Here's how the part is built. I have some questions about the finished solid (model axes, mm). A direction names the side the tool comes from. Give positions to 0.01 mm unless a question says otherwise; leave off trailing zeros. Loops run counter-clockwise (first coordinate to the right, second up) from the corner with the lowest first, then second, coordinate; pieces in that order, holes last. Notation, with made-up numbers: (-14, 79.5) - (12, 79.5) arc R35 cw to (12, 113.5) - close; hole circle Ø4 at (80, -21). An arc over 180 degrees is marked (long way). Use one line per item in the form item = value.
from build123d import *

# Parameters (mm, degrees)
BOSS_EXTRUDE1_DEPTH      = 5
BOSS_EXTRUDE1_DEPTH_BACK = 5
SKETCH1_R                = 1.75
SKETCH4_R                = 5.3
SKETCH4_R_2              = 1.75
BOSS_EXTRUDE2_DEPTH      = 1
M3_CLEARANCE_HOLE1_D     = 3.6


with BuildPart() as part:
    # Sketch1 → Boss-Extrude1 (new, two sides: drawn at the far end of the back side and taken through both)
    with BuildSketch(Plane.XY.offset(-BOSS_EXTRUDE1_DEPTH_BACK)):
        with BuildLine():
            Line((-29.2, 10.8), (-30.316718427, 10.8))
            ThreePointArc((-30.316718427, 10.8), (-35.8, 10), (-30.316718427, 9.2))
            Line((-30.316718427, 9.2), (-29.2, 9.2))
            Line((-29.2, 9.2), (-29.2, 10.8))
        make_face()
        with Locations(Location((-33, 10, 0), (0, 0, 180))):
            Circle(SKETCH1_R, mode=Mode.SUBTRACT)
    extrude(amount=BOSS_EXTRUDE1_DEPTH + BOSS_EXTRUDE1_DEPTH_BACK)

    # Sketch4 → Boss-Extrude2 (add)
    with BuildSketch(Plane.XY.offset(5)):
        with Locations((-33, 10)):
            Circle(SKETCH4_R)
        with Locations((-33, 10)):
            Circle(SKETCH4_R_2, mode=Mode.SUBTRACT)
    extrude(amount=BOSS_EXTRUDE2_DEPTH)

    # M3 Clearance Hole1 (through all)
    with Locations(Plane.XY.offset(6)):
        with Locations((-33, 10)):
            Hole(M3_CLEARANCE_HOLE1_D / 2)


solid = part.part
(1) If I drill on probe 1 along Y at (x, z) = (-33, 0); probe 2 along Z at (x, y) = (-36.25, 6.25); probe 3 along X at (y, z) = (11.5, -1.5), over which ranges is the centre line in solid material (lowest first)?
Geometry says:
probe_1 = 7.2 to 8.2, 11.8 to 12.8
probe_2 = 5 to 6
probe_3 = -35.36 to -33.99, -32.01 to -30.64
(2) If we section it at C-C (z = -0.25): List the corners of the cut face in (x, y) for me.
Geometry says:
outline = (-30.32, 9.2) - (-29.2, 9.2) - (-29.2, 10.8) - (-30.32, 10.8) arc R2.8 ccw (long way) to start; hole circle Ø3.6 at (-33, 10)
(3) If we section it at A-A (y = 10): List the corners of the cut face in (x, z) for me, plus the area to 3 significant figures.
Geometry says:
outline = (-38.3, 5) - (-35.8, 5) - (-35.8, -5) - (-34.8, -5) - (-34.8, 6) - (-38.3, 6) - close; (-31.2, -5) - (-29.2, -5) - (-29.2, 5) - (-27.7, 5) - (-27.7, 6) - (-31.2, 6) - close
area = 37.0 mm²
(4) Thinking about a two-plate mould opening in Y: for faces 6 (the cylindrical face through (-34.663, 9.311, 0.423)), 7 (the cylindrical face through (-28.104, 7.97, 5.493)), 8 (the flat face through (-30.7, 7.7, 5)), which applies, pulls with the +Y half, pulls with the -Y half, needs draft (parallel to the pull), parting line crosses it, or undercut?
Geometry says:
face_6 = undercut
face_7 = parting line crosses it
face_8 = needs draft
(5) For faces 1 (the cylindrical face through (-35.8, 10.1, -0.1)), 2 (the flat face through (-33, 8, 6)), 3 (the flat face through (-29.2, 10, 0)), 4 (the flat face through (-30, 10.8, 0)), 5 (the flat face through (-30, 9.2, 0)), which set-ups out of +Z, -Z, +X, -X, +Y, -Y let a thin tool reach every point of the face, with its end or its side?
Geometry says:
face_1 = -Z
face_2 = +Z, +X, -X, +Y, -Y
face_3 = -Z, +X, +Y, -Y
face_4 = -Z, +X, +Y
face_5 = -Z, +X, -Y
(6) If we section it at D-D (y = 7.75): List the corners of the cut face in (x, z) for me, plus the area to 3 significant figures.
Geometry says:
outline = (-37.8, 5) - (-34.67, 5) - (-34.67, -5) - (-31.33, -5) - (-31.33, 5) - (-28.2, 5) - (-28.2, 6) - (-37.8, 6) - close
area = 42.9 mm²
(7) For P1, Ø1.8, axis at y = 10.5, z = 2, coming from the +X side; P2, Ø6, axis at y = 11.5, z = 1.5, coming from the -X side; P3, Ø4, axis at x = -35, y = 12, coming from the -Z side; P4, Ø1.5, axis at x = -29.5, z = 0, coming from the +Y side, each with a flat end and sliding along its axis, tell me the tip position at first contact or that it passes through.
Geometry says:
P1 = -29.2
P2 = -35.8
P3 = -5
P4 = 10.8
(8) If we section it at B-B (x = -33): List the corners of the cut face in (y, z) for me, plus the area to 3 significant figures.
Geometry says:
outline = (4.7, 5) - (7.2, 5) - (7.2, -5) - (8.2, -5) - (8.2, 6) - (4.7, 6) - close; (11.8, -5) - (12.8, -5) - (12.8, 5) - (15.3, 5) - (15.3, 6) - (11.8, 6) - close
area = 27.0 mm²
